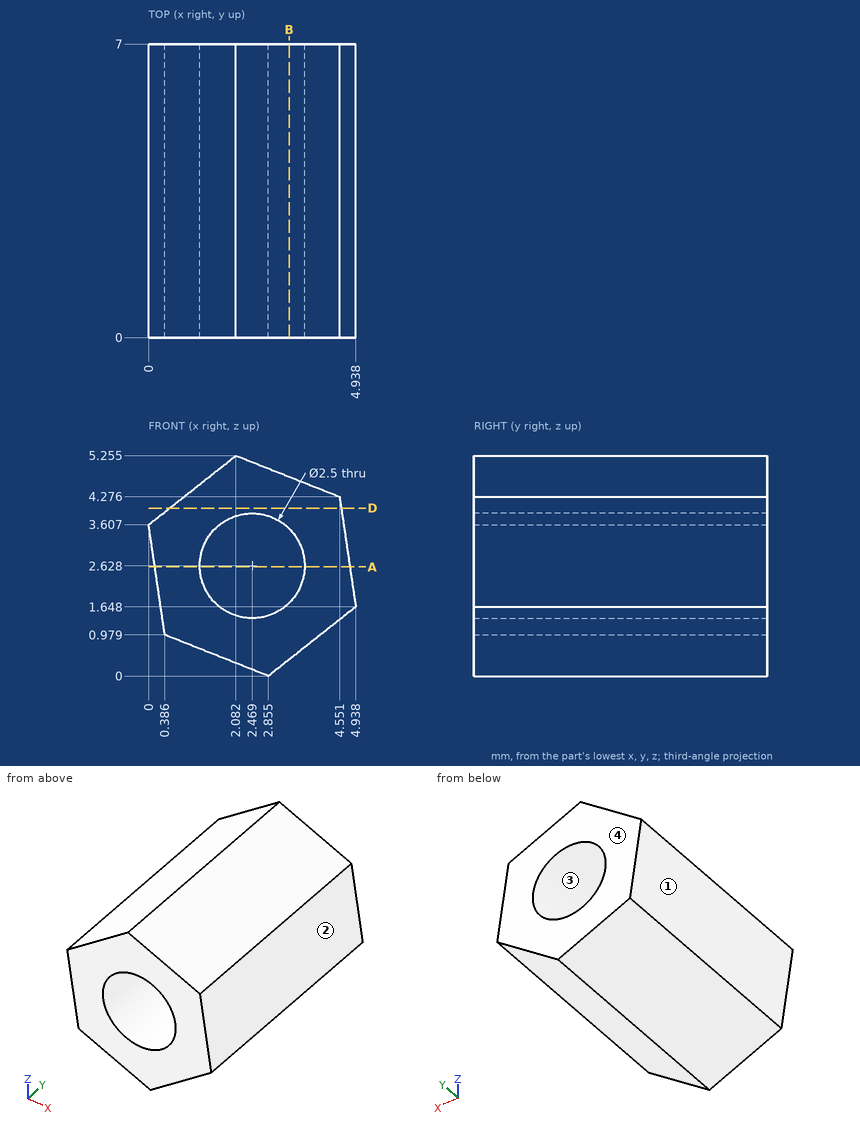
Study the drawing (mm; zero at the part's minimum x, y, z) and answer. Round coordinates to 2 decimals unless told otherwise and drop trailing zeros. Write each loop counter-clockwise with the first axis right and the second up, starting at its lowest first coordinate (ties: lowest second). Pieces come first, ordered by that corner, then holes. Notation, with made-up numbers: (7.5, 80.5) - (55.5, 80.5) arc R23 ccw to (55.5, 97.5) - close; hole circle Ø5 at (-21, 87.5). An arc over 180 degrees is marked (long way). Use CSV: the item, a comma, the result in double quotes.
Q1. Find section B-B, the plane x = 3.35. Write down the section's boundary in (y, z) (1 decimal), then the cut area to 3 significant figures.
Values:
outline,"(0, 0.4) - (7, 0.4) - (7, 1.7) - (0, 1.7) - close; (0, 3.5) - (7, 3.5) - (7, 4.8) - (0, 4.8) - close"
area,"18.1 mm²"
Q2. Determine the mould class of the marked faces 1, 2, 3 and 4 for opening direction X: +X half, -X half, draft (parallel to the pull), parting line (faces both ways), or undercut.
Values:
face 1,"-X half"
face 2,"+X half"
face 3,"undercut"
face 4,"draft"
Q3. Straight lines are drawn through the part: line 1 along Z through (x, y) = (2.7, 1) (1 decimal); line 2 along Z through (x, y) = (1.85, 1) (1 decimal); line 3 along X through (y, z) = (6.25, 3.75) (1 decimal). For each, find the intervals that lie inside material, in ascending order.
Values:
line 1,"z = 0.1 to 1.4, 3.9 to 5"
line 2,"z = 0.4 to 1.5, 3.7 to 5.1"
line 3,"x = 0.2 to 1.9, 3 to 4.6"
Q4. Find section D-D, the plane z = 4. Write down the section's boundary in (x, y).
Values:
outline,"(0.5, 0) - (4.59, 0) - (4.59, 7) - (0.5, 7) - close"
Q5. Find section A-A, the plane z = 2.6. Write down the section's boundary in (x, y).
Values:
outline,"(0.15, 0) - (1.22, 0) - (1.22, 7) - (0.15, 7) - close; (3.72, 0) - (4.8, 0) - (4.8, 7) - (3.72, 7) - close"
